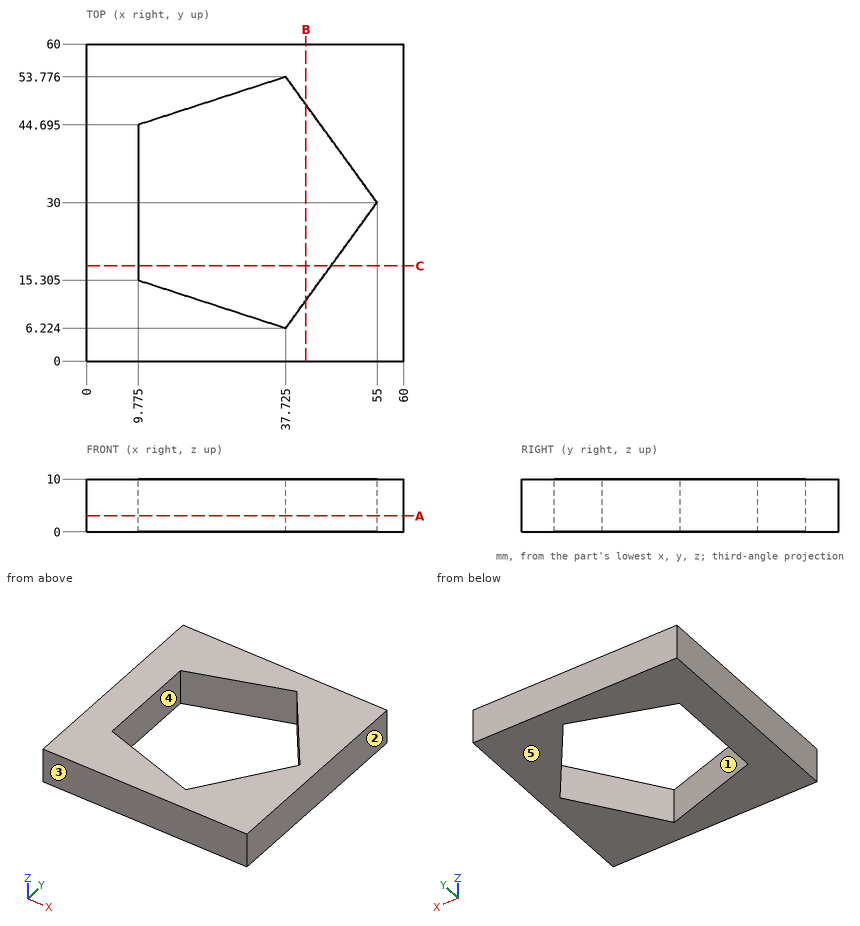
Geometry: see drawing. Coordinates: mm, zero at the bounding-box minimum. A direction names the side the tool comes from. Coordinates: 2 decimals unless noted, no trailing zeros. Loops run counter-clockwise (first coordinate to the right, second up) from the corner with the lowest first, then second, coordinate; pieces in that order, holes last. Notation, with made-up numbers: (8.25, 59) - (40.25, 59) arc R34 ccw to (40.25, 93) - close; hole circle Ø6 at (47.5, -4.5). An arc over 180 degrees is marked (long way). Put each result on its own line as item: value. Start each with the question number.
Q1. Cut plane C-C, the plane y = 18. Return loops of the section in (x, z) (1 decimal).
Q2. Line query: line 1 (Y direction, x = 23.5, z = 6.25) (1 decimal); line 2 (X direction, y = 17, z = 5.25) (1 decimal); line 3 (Y direction, x = 17, z = 9). Output: solid intervals per line, ascending.
Q3. Pull-direction query (Y, two-part tool) for the marked faces 3, 4 and 5; classes: released by +Y, released by -Y, zero draft, split by the parting line, or undercut.
Q4. Cut plane A-A, the plane z = 3. Return loops of the section in (x, y) (1 decimal).
Q5. Set-up query: the marked faces 1 and 2. Return all of +Z, -Z, +X, -X, +Y, -Y with unobstructed straight access to the full face (end or side cutting, diameter ignored); none if empty.
Q6. Cut plane B-B, the plane x = 41.5. Return loops of the section in (y, z), and give its area (3 significant figures).
Filled sheet:
1. outline: (0, 0) - (9.8, 0) - (9.8, 10) - (0, 10) - close; (46.3, 0) - (60, 0) - (60, 10) - (46.3, 10) - close
2. line 1: 0 to 10.8, 49.2 to 60
2. line 2: 0 to 9.8, 45.6 to 60
2. line 3: 0 to 12.96, 47.04 to 60
3. face 3: released by -Y
3. face 4: undercut
3. face 5: zero draft
4. outline: (0, 0) - (60, 0) - (60, 60) - (0, 60) - close; hole (9.8, 15.3) - (37.7, 6.2) - (55, 30) - (37.7, 53.8) - (9.8, 44.7) - close
5. face 1: +Z, -Z
5. face 2: +Z, -Z, +X, +Y, -Y
6. outline: (0, 0) - (11.42, 0) - (11.42, 10) - (0, 10) - close; (48.58, 0) - (60, 0) - (60, 10) - (48.58, 10) - close
6. area: 228 mm²
